```python
from build123d import *

# Parameters (mm, degrees)
SKETCH1_R           = 3.1115
BOSS_EXTRUDE1_DEPTH = 82.55
CHAMFER1_SIZE       = 0.508
FILLET1_R           = 0.381


with BuildPart() as part:
    # Sketch1 → Boss-Extrude1 (new body)
    with BuildSketch(Plane(origin=(0, 0, 0), x_dir=(0, 0, -1), z_dir=(1, 0, 0))):
        Circle(SKETCH1_R)
    extrude(amount=BOSS_EXTRUDE1_DEPTH)

    # Chamfer1
    chamfer1_edges = [part.edges().sort_by_distance(p)[0] for p in [
        (0, 0, 3.1115),
        (82.55, 0, 3.1115),
    ]]
    chamfer(chamfer1_edges, length=CHAMFER1_SIZE)

    # Fillet1
    fillet1_edges = [part.edges().sort_by_distance(p)[0] for p in [
        (82.55, 0, 2.6035),
        (0.508, 0, 3.1115),
        (82.042, 0, 3.1115),
        (0, 0, 2.6035),
    ]]
    fillet(fillet1_edges, radius=FILLET1_R)


solid = part.part
```
Build history of the part. All positions in model axes, mm. Coordinates: 2 decimals unless noted, no trailing zeros. Order: outer loops, then holes, each group sorted by start corner. A loop starts at its lowest first (then second) coordinate and runs counter-clockwise, first axis right, second up. Notation, with made-up numbers: M -9,19 L 16,19 A20 ccw 16,30 Z; hole C 8.5,3 d8. An arc over 180 degrees is marked long. One line per question, with ' | ' between items. Start each with the question number.
1. Flat gauge pins, fed straight in: P1, Ø2, axis at y = 2.5, z = -2, coming from the +X side; P2, Ø1, axis at x = 61, y = 1, coming from the -Z side. Where does each tip first touch, or does it go through?
2. Cut at A-A (x = 26). Write the cut outline in (y, z).
3. Wall check: line 1 along Y through (x, z) = (16, 1.5); line 2 along X through (y, z) = (-1.5, -2). Give the ranges that are in metal, low to high. Write a range as [from, to].
The answers:
1) P1: stops at x = 82.55 | P2: stops at z = -3.07
2) outline: C 0,0 d6.22
3) line 1: y = [-2.73, 2.73] | line 2: x = [0, 82.55]
